For this review, take the finished solid that the model builds, in its own axes (mm). A direction names the side the tool comes from. Coordinates: 2 decimals unless noted, no trailing zeros. Write each loop counter-clockwise with the first axis right and the second up, starting at its lowest first coordinate (ties: lowest second). Pieces come first, ordered by that corner, then holes. Notation, with made-up numbers: (-30.75, 77.5) -> (10.25, 77.5) arc R22 cw to (10.25, 98.5) -> close; hole circle Ø11 at (-3, 27.5). An arc over 180 degrees is marked (long way). Put each result on its own line as item: value. Start each with the question number.
Item 1: To check wall thickness, follow L1, parallel to X at y = 3.5, z = 14; L2, parallel to Y at x = -14, z = 16.25; L3, parallel to X at y = 9.5, z = 14. State the ranges of each line that lie inside material, in increasing order.
Item 2: Consider section C-C on y = 0. Give the boundary of the cut face in (x, z).
Item 3: Consider section B-B on z = 1.5. Give the boundary of the cut face in (x, y).
Item 4: Consider section A-A on x = 14. Give the boundary of the cut face in (y, z), and give its area (3 significant figures).
Item 5: Consider section D-D on z = 14.75. Give the boundary of the cut face in (x, y).
Item 6: For faces 4 (the cylindrical face through (24, 3.2, 16.8)), 5 (the flat face through (-1, 15, 0)), list the 3-axis set-ups (+Z, -Z, +X, -X, +Y, -Y) from which the entire face can be reached by the end or side of a thin tool; tool diameter is ignored.
Item 7: Insertion check: P1, Ø6.5, axis at x = -12, y = -1.5, coming from the +Z side; P2, Ø2, axis at x = -5.5, y = -6, coming from the -Z side; P3, Ø4, axis at x = 1.5, y = -4, coming from the -Z side. Each pin has a flat end and moves straight along its axis. Give the tip position at first contact, or say it passes through.
Item 8: The part is to be moulded in two halves that separate along Y. For faces 1 (the flat face through (-1, -16.5, 10)), 2 (the flat face through (-1, -15, 0)), 3 (the cylindrical face through (-4, 3.2, 16.8)), say which applies: +Y half, -Y half, draft (parallel to the pull), parting line (faces both ways), or undercut.
```python
from build123d import *

# Parameters (mm, degrees)
F0_W     = 73
F0_H     = 33
F1_DEPTH = 20
F2_R     = 10.5
F3_DEPTH = 6.5
F5_DEPTH = 73.001
F6_R     = 0.5


with BuildPart() as f1:
    # F0 (on Top) → F1 (new body)
    with BuildSketch(Plane.XY):
        Rectangle(F0_W, F0_H)
    extrude(amount=F1_DEPTH)

    # F2 (on face) → F3 (cut)
    with BuildSketch(Plane.XY.offset(20)):
        with Locations((-14, 0)):
            Circle(F2_R)
        with Locations((14, 0)):
            Circle(F2_R)
    extrude(amount=-F3_DEPTH, mode=Mode.SUBTRACT)

    # F4 (on face) → F5 (cut, through all)
    with BuildSketch(Plane.YZ.offset(36.5)):
        with BuildLine():
            Line((-12.541531007, 0), (12.541531007, 0))
            ThreePointArc((12.541531007, 0), (0, 10.7), (-12.541531007, 0))
        make_face()
        with BuildLine():
            ThreePointArc((-12.541531007, 0), (-1.0031341413, -14.6603207659), (12.7, -2))
            ThreePointArc((12.7, -2), (12.6603207659, -0.9968658587), (12.541531007, 0))
            Line((12.541531007, 0), (-12.541531007, 0))
        make_face()
    extrude(amount=-F5_DEPTH, mode=Mode.SUBTRACT)

    # F6
    f6_edges = [f1.edges().sort_by_distance(p)[0] for p in [
        (0, 16.5, 20),
        (0, -16.5, 20),
        (0, -12.541531, 0),
        (0, 12.541531, 0),
    ]]
    fillet(f6_edges, radius=F6_R)


solid = f1.part
```
Return value:
1. L1: -36.5 to -23.9, -4.1 to 4.1, 23.9 to 36.5
1. L2: -16.5 to -10.5, 10.5 to 16.5
1. L3: -36.5 to -18.47, -9.53 to 9.53, 18.47 to 36.5
2. outline: (-36.5, 10.7) -> (36.5, 10.7) -> (36.5, 20) -> (24.5, 20) -> (24.5, 13.5) -> (3.5, 13.5) -> (3.5, 20) -> (-3.5, 20) -> (-3.5, 13.5) -> (-24.5, 13.5) -> (-24.5, 20) -> (-36.5, 20) -> close
3. outline: (-36.5, -16.5) -> (36.5, -16.5) -> (36.5, -12.21) -> (-36.5, -12.21) -> close; (-36.5, 12.21) -> (36.5, 12.21) -> (36.5, 16.5) -> (-36.5, 16.5) -> close
4. outline: (-16.5, 0) -> (-12.96, 0) arc R0.5 ccw to (-12.47, 0.41) arc R12.7 cw to (12.47, 0.41) arc R0.5 ccw to (12.96, 0) -> (16.5, 0) -> (16.5, 19.5) arc R0.5 ccw to (16, 20) -> (10.5, 20) -> (10.5, 13.5) -> (-10.5, 13.5) -> (-10.5, 20) -> (-16, 20) arc R0.5 ccw to (-16.5, 19.5) -> close
4. area: 321 mm^2
5. outline: (-36.5, -16.5) -> (36.5, -16.5) -> (36.5, 16.5) -> (-36.5, 16.5) -> close; hole circle Ø21 at (-14, 0); hole circle Ø21 at (14, 0)
6. face 4: +Z
6. face 5: -Z, +X, -X, +Y, -Y
7. P1: z = 13.5
7. P2: z = 8.6
7. P3: z = 9.19
8. face 1: -Y half
8. face 2: draft
8. face 3: undercut
